```python
from build123d import *

# Parameters (mm, degrees)
SKETCH1_R                      = 12.75
BOSS_EXTRUDE1_DEPTH            = 5
F_6_0MM_DOWEL_HOLE1_D          = 4
SKETCH2_R                      = 6
BOSS_EXTRUDE2_DEPTH            = 20
SKETCH5_R                      = 9.85
BOSS_EXTRUDE3_DEPTH            = 20
F_6_0MM_DOWEL_HOLE2_D          = 12
F_6_0MM_DOWEL_HOLE3_D          = 3.5
F_6_0MM_DOWEL_HOLE3_DEPTH      = 20
SKETCH17_W                     = 1.75
SKETCH17_H                     = 5
F_6_0MM_DOWEL_HOLE4_AT_2_COUNT = 2
F_6_0MM_DOWEL_HOLE4_AT_2_PITCH = 10.946012973


with BuildPart() as part:
    # Sketch1 → Boss-Extrude1 (new body)
    with BuildSketch(Plane(origin=(0, 0, 0), x_dir=(1, 0, 0), z_dir=(0, 1, 0))):
        with Locations(Location((0, 0, 0), (0, 0, 270))):
            Circle(SKETCH1_R)
    extrude(amount=BOSS_EXTRUDE1_DEPTH)

    # Ø6.0mm Dowel Hole1 (through all)
    with Locations(Plane(origin=(0, 5, 0), x_dir=(1, 0, 0), z_dir=(0, 1, 0))):
        with Locations((-9.5, 0), (4.75, -8.227241336), (4.75, 8.227241336)):
            Hole(F_6_0MM_DOWEL_HOLE1_D / 2)

    # Sketch2 → Boss-Extrude2 (add)
    with BuildSketch(Plane(origin=(0, 5, 0), x_dir=(1, 0, 0), z_dir=(0, 1, 0))):
        with Locations(Location((0, 0, 0), (0, 0, 270))):
            Circle(SKETCH2_R)
    extrude(amount=BOSS_EXTRUDE2_DEPTH)

    # Sketch5 → Boss-Extrude3 (add)
    with BuildSketch(Plane(origin=(0, 25, 0), x_dir=(1, 0, 0), z_dir=(0, 1, 0))):
        with Locations(Location((0, 0, 0), (0, 0, 270))):
            Circle(SKETCH5_R)
    extrude(amount=BOSS_EXTRUDE3_DEPTH)

    # Ø6.0mm Dowel Hole2 (through all)
    with Locations(Plane(origin=(0, 45, 0), x_dir=(1, 0, 0), z_dir=(0, 1, 0))):
        with Locations((3, 0)):
            Hole(F_6_0MM_DOWEL_HOLE2_D / 2)

    # Ø6.0mm Dowel Hole3
    with Locations(Plane(origin=(0, 45, 0), x_dir=(1, 0, 0), z_dir=(0, 1, 0))):
        with Locations((-5.473006486, 5.473006486), (-5.473006486, -5.473006486)):
            Hole(F_6_0MM_DOWEL_HOLE3_D / 2, depth=F_6_0MM_DOWEL_HOLE3_DEPTH)

    # Sketch17 → Ø6.0mm Dowel Hole4 (revolve, cut)
    with BuildSketch(Plane(origin=(-5.473006486, 5, 5.473006486), x_dir=(0, 0, 1), z_dir=(1, 0, 0))):
        with Locations((0.875, 2.5)):
            Rectangle(SKETCH17_W, SKETCH17_H)
    f_6_0mm_dowel_hole4 = revolve(axis=Axis((-5.473006486, 11.35, 5.473006486), (0, -1, 0)), mode=Mode.SUBTRACT)

    # Ø6.0mm Dowel Hole4 at 2: Ø6.0mm Dowel Hole4 ×2
    with Locations(*[(0, 0, -i * F_6_0MM_DOWEL_HOLE4_AT_2_PITCH) for i in range(1, F_6_0MM_DOWEL_HOLE4_AT_2_COUNT)]):
        add(f_6_0mm_dowel_hole4, mode=Mode.SUBTRACT)


solid = part.part
```
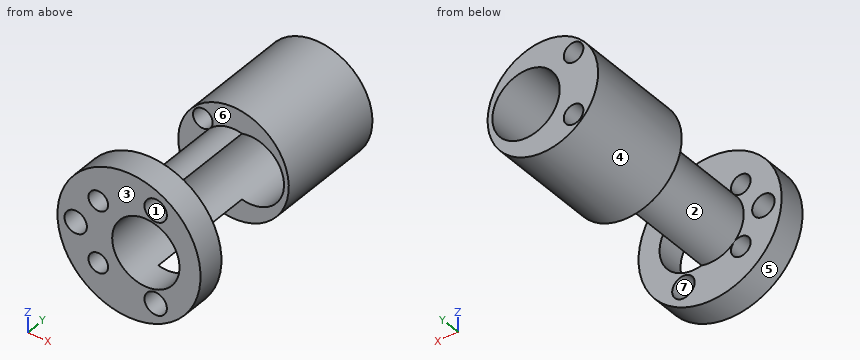
For this review, take the finished solid that the model builds, in its own axes (mm). Face numbers are marked on the shaded views. A direction names the side the tool comes from. Coordinates: 2 decimals unless noted, no trailing zeros. Order: outer loops, then holes, each group sorted by start corner. A loop starts at its lowest first (then second) coordinate and runs counter-clockwise, first axis right, second up. Notation, with made-up numbers: (36.5, 26.25) - (88.5, 26.25) arc R14 ccw to (88.5, 38.25) - close; hole circle Ø11 at (53.25, 17). An arc over 180 degrees is marked (long way). Answer as a JSON object with one key per item and string values. Group by question number.
1. The part is to be moulded in two halves that separate along X. For the marked faces 1, 2 and 3, say which applies: pulls with the +X half, pulls with the -X half, needs draft (parallel to the pull), parting line crosses it, or undercut.
2. We need section A-A on z = 0. State the section outline as (x, y) points, then the cut area to 4 significant figures.
3. We need section B-B on x = 0. State the section outline as (y, z) points, then the cut area to 3 significant figures.
4. Clearance check with flat-ended pins moving along their axes: P1, Ø1, axis at y = 38.5, z = -8.5, coming from the +X side; P2, Ø5, axis at y = 8.5, z = -9.5, coming from the -X side; P3, Ø4, axis at y = 24.5, z = 8, coming from the +X side; P4, Ø6, axis at y = 22.5, z = -4.5, coming from the -X side. State where each tip first meets the part, or that it passes through.
5. For the marked faces 4, 5, 6 and 7, list the 3-axis set-ups (+Z, -Z, +X, -X, +Y, -Y) from which the entire face can be reached by the end or side of a thin tool; tool diameter is ignored.
6. We need section C-C on z = 2.75. State the section outline as (x, y) points, then the cut area to 3 significant figures.
7. For probe 1 along Y at (x, z) = (1.25, -8); probe 2 along X at (y, z) = (28, 4.5); probe 3 along Y at (x, z) = (3.25, -8.5), list the stretches that pass through material, from the lowest coordinate up.
8. We need section D-D on x = 4.75. State the section outline as (y, z) points, then the cut area to 3 significant figures.
Final values:
{
 "1": {"face 1": "undercut", "face 2": "parting line crosses it", "face 3": "needs draft"},
 "2": {"outline": "(-12.75, 0) - (-11.5, 0) - (-11.5, 5) - (-12.75, 5) - close; (-9.85, 25) - (-6, 25) - (-6, 5) - (-7.5, 5) - (-7.5, 0) - (-3, 0) - (-3, 45) - (-9.85, 45) - close; (9, 0) - (12.75, 0) - (12.75, 5) - (9, 5) - close; (9, 25) - (9.85, 25) - (9.85, 45) - (9, 45) - close", "area": "261.5 mm²"},
 "3": {"outline": "(0, -12.75) - (5, -12.75) - (5, -6) - (25, -6) - (25, -9.85) - (45, -9.85) - (45, -5.2) - (0, -5.2) - close; (0, 5.2) - (45, 5.2) - (45, 9.85) - (25, 9.85) - (25, 6) - (5, 6) - (5, 12.75) - (0, 12.75) - close", "area": "294 mm²"},
 "4": {"P1": "x = 5.75", "P2": "through", "P3": "x = 7.76", "P4": "x = -9.43"},
 "5": {"face 4": "+Y", "face 5": "+Y, -Y", "face 6": "none", "face 7": "-Y"},
 "6": {"outline": "(-12.45, 0) - (-2.33, 0) - (-2.33, 45) - (-9.46, 45) - (-9.46, 25) - (-5.33, 25) - (-5.33, 5) - (-12.45, 5) - close; (8.33, 0) - (12.45, 0) - (12.45, 5) - (8.33, 5) - close; (8.33, 25) - (9.46, 25) - (9.46, 45) - (8.33, 45) - close", "area": "296 mm²"},
 "7": {"probe 1": "0 to 5, 25 to 45", "probe 2": "-8.76 to -6.93, -4.02 to -0.97, 6.97 to 8.76", "probe 3": "25 to 45"},
 "8": {"outline": "(0, -11.83) - (5, -11.83) - (5, -10.23) - (0, -10.23) - close; (0, -6.23) - (5, -6.23) - (5, -5.74) - (0, -5.74) - close; (0, 5.74) - (5, 5.74) - (5, 6.23) - (0, 6.23) - close; (0, 10.23) - (5, 10.23) - (5, 11.83) - (0, 11.83) - close; (25, -8.63) - (45, -8.63) - (45, -5.74) - (25, -5.74) - close; (25, 5.74) - (45, 5.74) - (45, 8.63) - (25, 8.63) - close", "area": "137 mm²"}
}
